from build123d import *

# Parameters (mm, degrees)
PAD007_DEPTH = 15


with BuildPart() as part:
    # Sketch007 → Pad007 (new body, symmetric)
    with BuildSketch(Plane.XY):
        with BuildLine():
            Line((-16.77051, -15), (-40, -15))
            Line((-40, -15), (-40, 0))
            Line((-40, 0), (40, 0))
            Line((40, 0), (40, -15))
            Line((40, -15), (16.77051, -15))
            ThreePointArc((16.77051, -15), (0, -2.5), (-16.77051, -15))
        make_face()
    extrude(amount=PAD007_DEPTH, both=True)

    # Sketch017 → Groove (revolve, cut)
    with BuildSketch(Plane(origin=(28, 0, 0), x_dir=(1, 0, 0), z_dir=(0, 0, 1))):
        Polygon((0, 0), (7.5, 0), (7.5, -7), (4.5, -10), (4.5, -27), (0, -27), align=None)
    revolve(axis=Axis((28, 0, 0), (0, 1, 0)), mode=Mode.SUBTRACT)

    # Sketch018 → Groove001 (revolve, cut)
    with BuildSketch(Plane(origin=(-28, 0, 0), x_dir=(1, 0, 0), z_dir=(0, 0, 1))):
        Polygon((0, 0), (7.5, 0), (7.5, -7), (4.5, -10), (4.5, -30), (0, -30), align=None)
    revolve(axis=Axis((-28, 0, 0), (0, 1, 0)), mode=Mode.SUBTRACT)


with BuildPart() as part_1:
    # Body007 placement: moved
    add(part.part.moved(Location((0, -30, 0))))


solid = part_1.part
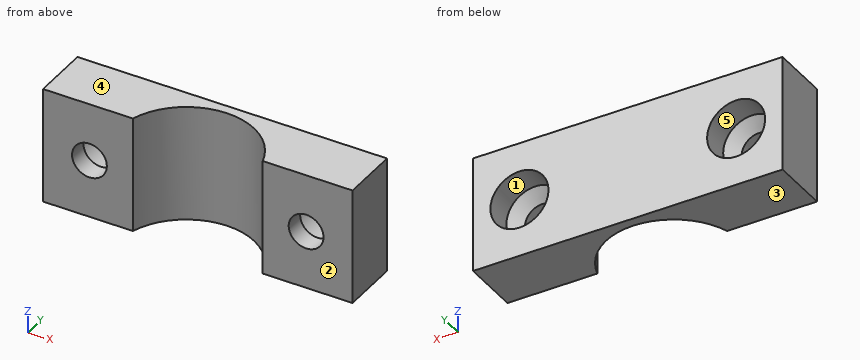
For this review, take the finished solid that the model builds, in its own axes (mm). Face numbers are marked on the shaded views. A direction names the side the tool comes from. Round coordinates to 2 decimals unless told otherwise and drop trailing zeros. Write each loop counter-clockwise with the first axis right and the second up, starting at its lowest first coordinate (ties: lowest second). Pieces come first, ordered by that corner, then holes. Notation, with made-up numbers: (45.5, 10) -> (81.5, 10) arc R34 cw to (81.5, 46) -> close; hole circle Ø5 at (59, 33.5). An arc over 180 degrees is marked (long way). Put each result on its own line as item: value.
Q1. Clearance check with flat-ended pins moving along their axes: pin 1 Ø10.5 at (x, z) = (28, 0) entering from +Y; pin 2 Ø12 at (x, z) = (-28, 0) entering from +Y; pin 3 Ø8 at (x, z) = (-13, -5.5) entering from -Y. State where each tip first meets the part, or that it passes through.
Determined:
pin 1: stops at y = -39.25
pin 2: stops at y = -38.5
pin 3: stops at y = -45
Q2. Consider section B-B on x = 28. State the section outline as (y, z) points, and give its area (3 significant figures).
Determined:
outline: (-45, -15) -> (-30, -15) -> (-30, -7.5) -> (-37, -7.5) -> (-40, -4.5) -> (-45, -4.5) -> close; (-45, 4.5) -> (-40, 4.5) -> (-37, 7.5) -> (-30, 7.5) -> (-30, 15) -> (-45, 15) -> close
area: 264 mm^2
Q3. To check wall thickness, follow L1, parallel to X at y = -32, z = 0; L2, parallel to Z at x = 26.5, y = -39.75; L3, parallel to X at y = -38.5, z = 5. State the ranges of each line that lie inside material, in increasing order. Write a range as [from, to].
Determined:
L1: x = [-40, -35.5], [-20.5, 20.5], [35.5, 40]
L2: z = [-15, -4.51], [4.51, 15]
L3: x = [-40, -31.32], [-24.68, -13.19], [13.19, 24.68], [31.32, 40]
Q4. Consider section C-C on y = -42. State the section outline as (x, z) points.
Determined:
outline: (-40, -15) -> (-15.56, -15) -> (-15.56, 15) -> (-40, 15) -> close; (15.56, -15) -> (40, -15) -> (40, 15) -> (15.56, 15) -> close; hole circle Ø9 at (-28, 0); hole circle Ø9 at (28, 0)
Q5. Consider section A-A on z = 0. State the section outline as (x, y) points.
Determined:
outline: (-40, -45) -> (-32.5, -45) -> (-32.5, -40) -> (-35.5, -37) -> (-35.5, -30) -> (-40, -30) -> close; (-23.5, -45) -> (-16.77, -45) arc R17.5 cw to (16.77, -45) -> (23.5, -45) -> (23.5, -40) -> (20.5, -37) -> (20.5, -30) -> (-20.5, -30) -> (-20.5, -37) -> (-23.5, -40) -> close; (32.5, -45) -> (40, -45) -> (40, -30) -> (35.5, -30) -> (35.5, -37) -> (32.5, -40) -> close
Q6. Machinability: for the marked faces 1 and 2, which of the approach directions +Z, -Z, +X, -X, +Y, -Y give a long, thin tool a straight path to every point of the face, cutting with its end or side? Answer none if there is none.
Determined:
face 1: +Y
face 2: +Z, -Z, +X, -X, -Y
Q7. Consider section D-D on z = 12. State the section outline as (x, y) points.
Determined:
outline: (-40, -45) -> (-16.77, -45) arc R17.5 cw to (16.77, -45) -> (40, -45) -> (40, -30) -> (-40, -30) -> close
Q8. The part is to be moulded in two halves that separate along Z. For the marked faces 3, 4 and 5, say which applies: released by +Z, released by -Z, zero draft, split by the parting line, or undercut.
Determined:
face 3: released by -Z
face 4: released by +Z
face 5: undercut
